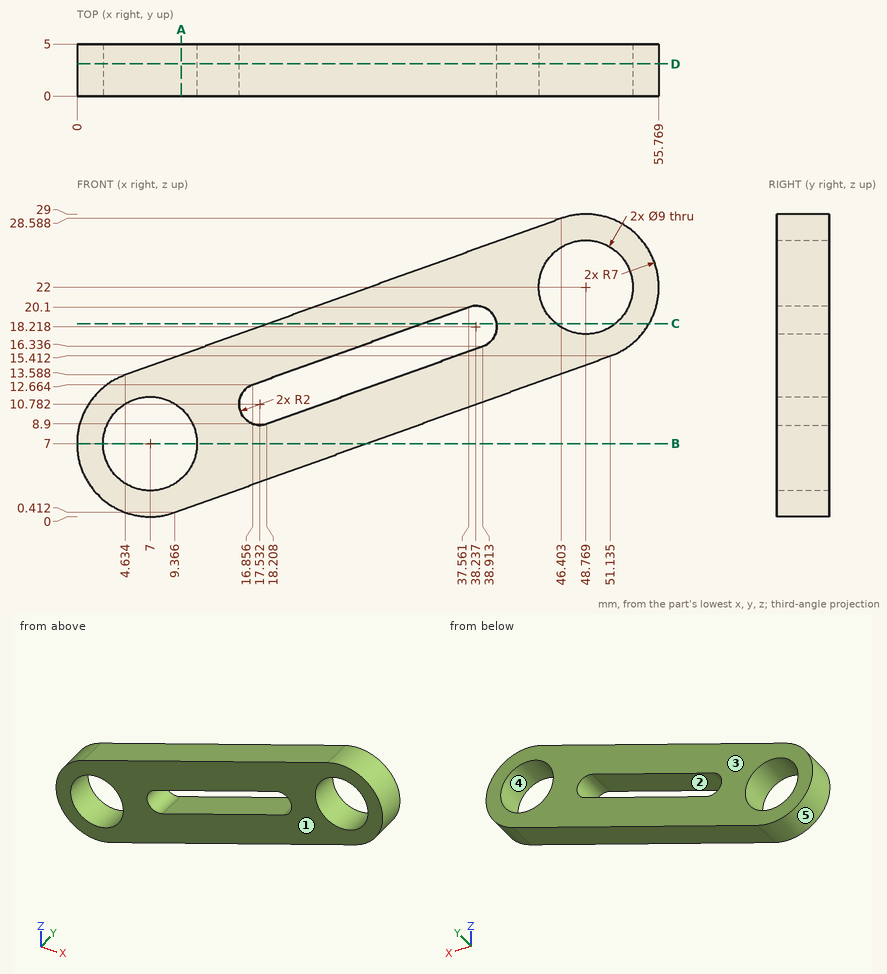
Design review of the part shown in the three views and the two pictorial views. Dimensions are in mm from the part's minimum x, y and z. A direction names the side the tool comes from. Give positions to 0.01 mm unless a question says otherwise; leave off trailing zeros. Write each loop counter-clockwise with the first axis right and the second up, starting at its lowest first coordinate (ties: lowest second). Pieces come first, ordered by that corner, then holes. Notation, with made-up numbers: M -7.75,62 L 48.25,62 A18 cw 48.25,91 Z; hole C 16.5,-16 d4. An arc over 180 degrees is marked long. Answer as CSV lines item,"result".
1. Consider section A-A, the plane x = 10. Write out the cut boundary in (y, z) (1 decimal).
Findings:
outline,"M 0,0.6 L 5,0.6 L 5,3.6 L 0,3.6 Z; M 0,10.4 L 5,10.4 L 5,15.5 L 0,15.5 Z"
2. Consider section B-B, the plane z = 7. Write out the cut boundary in (x, y).
Findings:
outline,"M 0,0 L 2.5,0 L 2.5,5 L 0,5 Z; M 11.5,0 L 27.71,0 L 27.71,5 L 11.5,5 Z"
3. Wall thickness on line 1 (Z direction, x = 21, y = 1.15) (1 decimal); line 2 (Z direction, x = 30.5, y = 2.3) (1 decimal): over which ranges is each line inside the solid? List them lowest first.
Findings:
line 1,"z = 4.6 to 9.9, 14.2 to 19.5"
line 2,"z = 8 to 13.3, 17.6 to 22.9"
4. For the marked faces 1 and 2, list the 3-axis set-ups (+Z, -Z, +X, -X, +Y, -Y) from which the entire face can be reached by the end or side of a thin tool; tool diameter is ignored.
Findings:
face 1,"+Z, -Z, +X, -X, -Y"
face 2,"+Y, -Y"
5. Consider section D-D, the plane y = 3.1. Write out the cut boundary in (x, z) (1 decimal).
Findings:
outline,"M 4.6,13.6 A7 ccw 9.4,0.4 L 51.1,15.4 A7 ccw 46.4,28.6 Z; hole C 7,7 d9; hole M 16.9,12.7 A2 ccw 18.2,8.9 L 38.9,16.3 A2 ccw 37.6,20.1 Z; hole C 48.8,22 d9"
6. Draft analysis for pull direction Z (two halves, no side actions). For the marked faces 3, 4 and 5, state which applies: +Z half, -Z half, draft (parallel to the pull), parting line (faces both ways), or undercut.
Findings:
face 3,"draft"
face 4,"undercut"
face 5,"parting line"
7. Consider section C-C, the plane z = 18.5. Write out the cut boundary in (x, y) (1 decimal), then the cut area to 3 significant figures.
Findings:
outline,"M 18.3,0 L 33.1,0 L 33.1,5 L 18.3,5 Z; M 40.2,0 L 45.9,0 L 45.9,5 L 40.2,5 Z; M 51.6,0 L 54.8,0 L 54.8,5 L 51.6,5 Z"
area,"119 mm2"
8. For pin 1 (1 mm diameter, centred on x = 12.5, y = 4.5, fed in from -Z), flat-tipped, find the tip position at first contact; note if it passes through.
Findings:
pin 1,"stops at z = 1.36"
